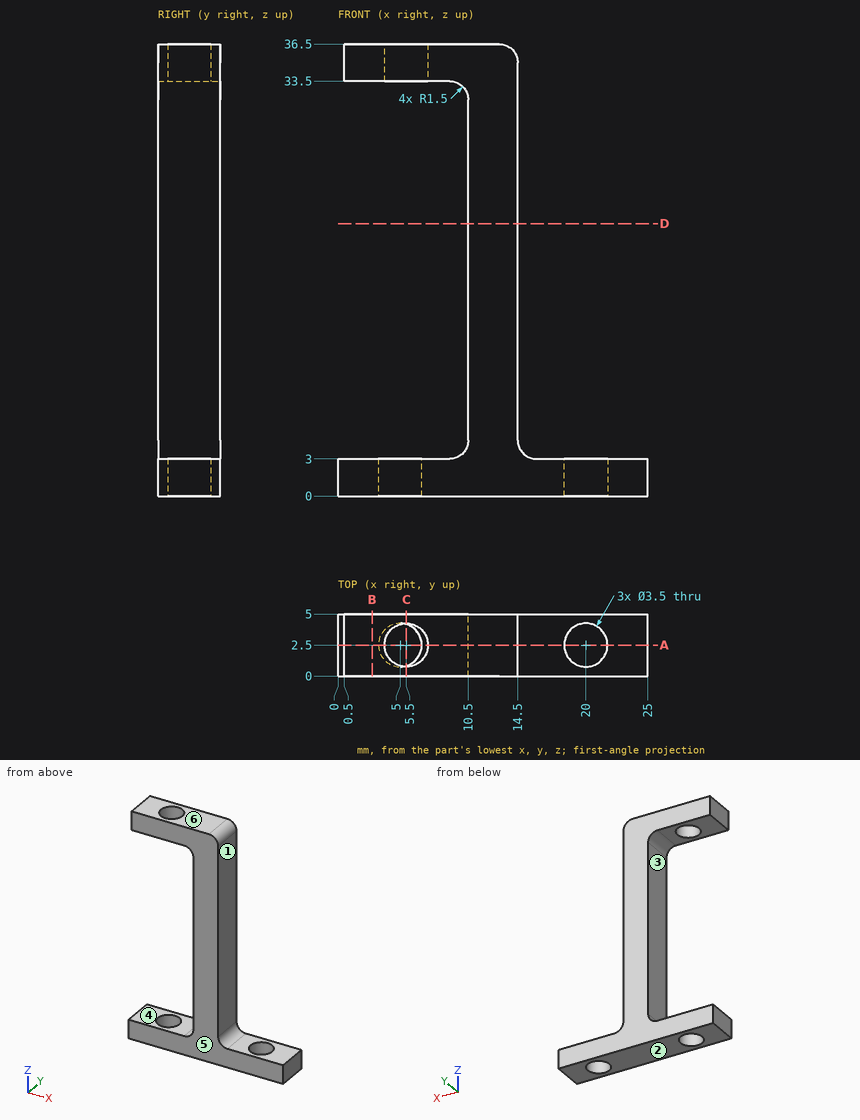
Here's the drawing with two shaded views (mm, measured from the low corner). I have some questions. A direction names the side the tool comes from. Coordinates: 2 decimals unless noted, no trailing zeros. Order: outer loops, then holes, each group sorted by start corner. A loop starts at its lowest first (then second) coordinate and runs counter-clockwise, first axis right, second up. Notation, with made-up numbers: (66, 22) - (73, 22) arc R11 ccw to (73, 27) - close; hole circle Ø8 at (43, 8.5). An arc over 180 degrees is marked (long way). Answer in a Markdown table with one row per item.
1. For pin 1 (1.5 mm diameter, centred on y = 2.5, z = 22, fed in from -X); pin 2 (1.5 mm diameter, centred on y = 2, z = 10.5, fed in from +X); pin 3 (3 mm diameter, centred on x = 5, y = 2.5, fed in from -Z), each with a flat end and sliding along its axis, tell me the tip position at first contact or that it passes through.
Reply:
| item | result |
|---|---|
| pin 1 | stops at x = 10.5 |
| pin 2 | stops at x = 14.5 |
| pin 3 | stops at z = 33.5 |
2. If we mould it in two halves opening along Z, with no side actions, what happens to the marked faces 4, 5 and 6? For each: pulls with the +Z half, pulls with the -Z half, needs draft (parallel to the pull), parting line crosses it, or undercut.
Reply:
| item | result |
|---|---|
| face 4 | undercut |
| face 5 | needs draft |
| face 6 | pulls with the +Z half |
3. Suppose I cut it at B-B (x = 2.75). Please give me the cut outline in (y, z), and give its area (3 significant figures).
Reply:
| item | result |
|---|---|
| outline | (0, 0) - (5, 0) - (5, 3) - (0, 3) - close; (0, 33.5) - (5, 33.5) - (5, 36.5) - (0, 36.5) - close |
| area | 30.0 mm^2 |
4. Suppose I cut it at C-C (x = 5.5). Please give me the cut outline in (y, z), and give its area (3 significant figures).
Reply:
| item | result |
|---|---|
| outline | (0, 0) - (0.82, 0) - (0.82, 3) - (0, 3) - close; (0, 33.5) - (0.75, 33.5) - (0.75, 36.5) - (0, 36.5) - close; (4.18, 0) - (5, 0) - (5, 3) - (4.18, 3) - close; (4.25, 33.5) - (5, 33.5) - (5, 36.5) - (4.25, 36.5) - close |
| area | 9.44 mm^2 |
5. If I drill on line 1 along Z through (x, y) = (1.25, 1.35); line 2 along X through (y, z) = (1.6, 2.5); line 3 along Z through (x, y) = (23, 3.4), over which ranges is the centre line in solid material (lowest first)?
Reply:
| item | result |
|---|---|
| line 1 | z = 0 to 3, 33.5 to 36.5 |
| line 2 | x = 0 to 3.5, 6.5 to 18.5, 21.5 to 25 |
| line 3 | z = 0 to 3 |
6. Suppose I cut it at D-D (z = 22). Please give me the cut outline in (x, y), and give its area (3 significant figures).
Reply:
| item | result |
|---|---|
| outline | (10.5, 0) - (14.5, 0) - (14.5, 5) - (10.5, 5) - close |
| area | 20.0 mm^2 |
7. Suppose I cut it at A-A (y = 2.5). Please give me the cut outline in (x, z), and give its area (3 significant figures).
Reply:
| item | result |
|---|---|
| outline | (0, 0) - (3.25, 0) - (3.25, 3) - (0, 3) - close; (0.5, 33.5) - (3.75, 33.5) - (3.75, 36.5) - (0.5, 36.5) - close; (6.75, 0) - (18.25, 0) - (18.25, 3) - (16, 3) arc R1.5 cw to (14.5, 4.5) - (14.5, 35) arc R1.5 ccw to (13, 36.5) - (7.25, 36.5) - (7.25, 33.5) - (9, 33.5) arc R1.5 cw to (10.5, 32) - (10.5, 4.5) arc R1.5 cw to (9, 3) - (6.75, 3) - close; (21.75, 0) - (25, 0) - (25, 3) - (21.75, 3) - close |
| area | 208 mm^2 |
8. For the marked faces 1, 2 and 3, which set-ups out of +Z, -Z, +X, -X, +Y, -Y let a thin tool reach every point of the face, with its end or its side?
Reply:
| item | result |
|---|---|
| face 1 | +Z, +X, +Y, -Y |
| face 2 | -Z, +X, -X, +Y, -Y |
| face 3 | -X, +Y, -Y |
